Autodesk Inventor part; units mm, degrees
ref_plane "YZ Plane" through (0, 0, 0) normal (1, 0, 0) x (0, 1, 0)
ref_plane "XZ Plane" through (0, 0, 0) normal (0, 1, 0) x (-1, 0, 0)
ref_plane "XY Plane" through (0, 0, 0) normal (0, 0, 1) x (1, 0, 0)
sketch "Sketch1" plane through (0, 0, 0) normal (0, 1, 0) x (-1, 0, 0)
  line L0 (0, 0) -> (304.8, 0)
  line L1 (304.8, 0) -> (304.8, 228.6)
  line L2 (304.8, 228.6) -> (0, 228.6)
  line L3 (0, 228.6) -> (0, 0)
  dimension "d0" = 228.6
  dimension "d1" = 304.8
extrude "Extrusion1" add sketch "Sketch1" along normal blind 6.35
sketch "Sketch2" plane through (0, 6.35, 0) normal (0, 1, 0) x (1, 0, 0)
  line L0 (0, -228.6) -> (0, 0)
  line L1 (0, -68.6) -> (-30, -68.6)
  line L2 (-30, -68.6) -> (-30, -143.6)
  line L3 (-30, -143.6) -> (0, -143.6)
  line L4 (0, -143.6) -> (0, -68.6)
  line L5 (-304.8, -228.6) -> (0, -228.6)
  dimension "d4" = 75
  dimension "d5" = 85
  dimension "d6" = 30
extrude "Extrusion2" cut sketch "Sketch2" against normal blind 10
properties part number "Board"
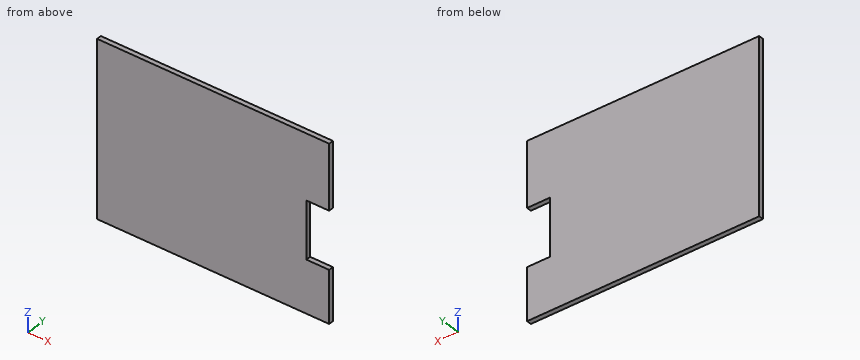
Can you work these out from the model? Positions are in its coordinate system, mm. Coordinates: 2 decimals unless noted, no trailing zeros. Write each loop counter-clockwise with the first axis right and the second up, starting at its lowest first coordinate (ties: lowest second). Pieces come first, ordered by that corner, then holes. Notation, with made-up numbers: (-29.5, 7.25) -> (27.5, 7.25) arc R36 ccw to (27.5, 45.25) -> close; hole circle Ø1 at (-11, 89.5). An arc over 180 degrees is marked (long way). Write item = value, one per line.
(1) Imagine slicing it at A-A (y = 2.75). Please give me the cut outline in (x, z).
Verdict:
outline = (-304.8, 0) -> (0, 0) -> (0, 68.6) -> (-30, 68.6) -> (-30, 143.6) -> (0, 143.6) -> (0, 228.6) -> (-304.8, 228.6) -> close
(2) For pin 1 (12 mm diameter, centred on x = -188.5, z = 49, fed in from -Y); pin 2 (1.9 mm diameter, centred on y = 3, z = 92.5, fed in from +X), each with a flat end and sliding along its axis, tell me the tip position at first contact or that it passes through.
Verdict:
pin_1 = 0
pin_2 = -30
(3) If I drill on probe 1 along Z at (x, y) = (-17.5, 5); probe 2 along X at (y, z) = (2.5, 115), over which ranges is the centre line in solid material (lowest first)?
Verdict:
probe_1 = 0 to 68.6, 143.6 to 228.6
probe_2 = -304.8 to -30
